from build123d import *
from OCP.BRepFilletAPI import BRepFilletAPI_MakeChamfer

# Parameters (mm, degrees)
ESQUISSE1_W             = 20
ESQUISSE1_H             = 34
BOSS_EXTRU_1_DEPTH      = 4
ESQUISSE2_W             = 8
ESQUISSE2_H             = 7
ENL_V_MAT_EXTRU_1_DEPTH = 21.124611797
CONG_1_R                = 4
ESQUISSE3_W             = 6
ESQUISSE3_H             = 34
BOSS_EXTRU_2_DEPTH      = 20
ESQUISSE4_R             = 2.1
ENL_V_MAT_EXTRU_2_DEPTH = 36.566838488
CHANFREIN1_SIZE         = 8
CHANFREIN1_SIZE2        = 4.618802154
CONG_2_R                = 4
ESQUISSE5_R             = 3.2
ENL_V_MAT_EXTRU_3_DEPTH = 29.08914381
ESQUISSE6_R             = 5.5
ENL_V_MAT_EXTRU_4_DEPTH = 29.08914381
ESQUISSE7_R             = 4
ENL_V_MAT_EXTRU_5_DEPTH = 3


with BuildPart() as part:
    # Esquisse1 → Boss.-Extru.1 (new body)
    with BuildSketch(Plane.XY):
        Rectangle(ESQUISSE1_W, ESQUISSE1_H)
    extrude(amount=BOSS_EXTRU_1_DEPTH)

    # Esquisse2 → Enlèv. mat.-Extru.1 (cut, through all)
    with BuildSketch(Plane.XY.offset(4)):
        with Locations((0, 13.5)):
            Rectangle(ESQUISSE2_W, ESQUISSE2_H)
        with Locations((0, -13.5)):
            Rectangle(ESQUISSE2_W, ESQUISSE2_H)
    extrude(amount=-ENL_V_MAT_EXTRU_1_DEPTH, mode=Mode.SUBTRACT)

    # Congé1
    cong_1_edges = [part.edges().sort_by_distance(p)[0] for p in [
        (0, -10, 4),
        (0, 10, 4),
    ]]
    fillet(cong_1_edges, radius=CONG_1_R - 0.0001)  # a hair under: the kernel refuses the full size

    # Esquisse3 → Boss.-Extru.2 (add)
    with BuildSketch(Plane.XY.offset(4)):
        with Locations((-7, 0)):
            Rectangle(ESQUISSE3_W, ESQUISSE3_H)
        with Locations((7, 0)):
            Rectangle(ESQUISSE3_W, ESQUISSE3_H)
    extrude(amount=BOSS_EXTRU_2_DEPTH)

    # Esquisse4 → Enlèv. mat.-Extru.2 (cut, through all)
    with BuildSketch(Plane(origin=(10, 0, 0), x_dir=(0, 0, -1), z_dir=(1, 0, 0))):
        with Locations(Location((-19, 9, 0), (0, 0, 90))):
            Circle(ESQUISSE4_R)
        with Locations(Location((-19, -9, 0), (0, 0, 90))):
            Circle(ESQUISSE4_R)
    extrude(amount=-ENL_V_MAT_EXTRU_2_DEPTH, mode=Mode.SUBTRACT)

    # Chanfrein1: one chamfer whose edges measure the first distance from different faces: ONE call of the kernel's chamfer builder (chamfer() names one face for all edges)
    chanfrein1_edges_1 = [part.edges().sort_by_distance(p)[0] for p in [
        (-7, -17, 24),
    ]]
    chanfrein1_side_1 = [part.faces().sort_by_distance(p)[0] for p in [
        (-7, -17, 12),
    ]]
    chanfrein1_edges_2 = [part.edges().sort_by_distance(p)[0] for p in [
        (-7, 17, 24),
    ]]
    chanfrein1_side_2 = [part.faces().sort_by_distance(p)[0] for p in [
        (-7, 17, 12),
    ]]
    chanfrein1_edges_3 = [part.edges().sort_by_distance(p)[0] for p in [
        (7, -17, 24),
    ]]
    chanfrein1_side_3 = [part.faces().sort_by_distance(p)[0] for p in [
        (7, -17, 12),
    ]]
    chanfrein1_edges_4 = [part.edges().sort_by_distance(p)[0] for p in [
        (7, 17, 24),
    ]]
    chanfrein1_side_4 = [part.faces().sort_by_distance(p)[0] for p in [
        (7, 17, 12),
    ]]
    chanfrein1 = BRepFilletAPI_MakeChamfer(part.part.solid().wrapped)
    for e in chanfrein1_edges_1:
        chanfrein1.Add(CHANFREIN1_SIZE, CHANFREIN1_SIZE2, e.wrapped, chanfrein1_side_1[0].wrapped)  # the first distance lies on this face
    for e in chanfrein1_edges_2:
        chanfrein1.Add(CHANFREIN1_SIZE, CHANFREIN1_SIZE2, e.wrapped, chanfrein1_side_2[0].wrapped)  # the first distance lies on this face
    for e in chanfrein1_edges_3:
        chanfrein1.Add(CHANFREIN1_SIZE, CHANFREIN1_SIZE2, e.wrapped, chanfrein1_side_3[0].wrapped)  # the first distance lies on this face
    for e in chanfrein1_edges_4:
        chanfrein1.Add(CHANFREIN1_SIZE, CHANFREIN1_SIZE2, e.wrapped, chanfrein1_side_4[0].wrapped)  # the first distance lies on this face
    add(Compound.cast(chanfrein1.Shape()), mode=Mode.REPLACE)

    # Congé2
    cong_2_edges = [part.edges().sort_by_distance(p)[0] for p in [
        (-7, 12.381197846, 24),
        (-7, -12.381197846, 24),
        (-7, -17, 16),
        (7, 12.381197846, 24),
        (7, -12.381197846, 24),
        (7, -17, 16),
        (-7, 17, 16),
        (7, 17, 16),
    ]]
    fillet(cong_2_edges, radius=CONG_2_R)

    # Esquisse5 → Enlèv. mat.-Extru.3 (cut, through all)
    with BuildSketch(Plane.XY.offset(4)):
        Circle(ESQUISSE5_R)
    extrude(amount=-ENL_V_MAT_EXTRU_3_DEPTH, mode=Mode.SUBTRACT)

    # Esquisse6 → Enlèv. mat.-Extru.4 (cut, through all)
    with BuildSketch(Plane.XY.offset(4)):
        Circle(ESQUISSE6_R)
    extrude(amount=ENL_V_MAT_EXTRU_4_DEPTH, mode=Mode.SUBTRACT)

    # Esquisse7 → Enlèv. mat.-Extru.5 (cut)
    with BuildSketch(Plane(origin=(10, 0, 0), x_dir=(0, 0, -1), z_dir=(1, 0, 0))):
        with Locations(Location((-19, 9, 0), (0, 0, 90))):
            Circle(ESQUISSE7_R)
        with Locations(Location((-19, -9, 0), (0, 0, 90))):
            Circle(ESQUISSE7_R)
    extrude(amount=-ENL_V_MAT_EXTRU_5_DEPTH, mode=Mode.SUBTRACT)


solid = part.part
Geometry check sheet. Reference: the model listing, model coordinates, mm. A direction names the side the tool comes from. Round coordinates to 2 decimals unless told otherwise and drop trailing zeros. Write each loop counter-clockwise with the first axis right and the second up, starting at its lowest first coordinate (ties: lowest second). Pieces come first, ordered by that corner, then holes. Notation, with made-up numbers: (-32, 46) -> (4, 46) arc R21 ccw to (4, 64) -> close; hole circle Ø5 at (47, -30.75). An arc over 180 degrees is marked (long way). One line per item, written item: value. Start each with the question number.
(1) Scan lines: line 1 (X direction, y = 8, z = 6.75); line 2 (Z direction, x = 8.55, y = -9); line 3 (X direction, y = -11.5, z = 21). Record each from-to range of solid material in increasing order. Write a range as [from, to].
(2) Go/stop test with flat-tipped pins: pin 1 Ø4 at (y, z) = (-9, 19.5) entering from +X; pin 2 Ø3 at (x, z) = (-2, 3) entering from -Y; pin 3 Ø4 at (x, z) = (-1.5, 19) entering from -Y; pin 4 Ø8.5 at (x, y) = (0, 0) entering from +Z. Record where each tip stops, or that it passes through.
(3) Cross-section at D-D, the plane y = 9. Record the cut outline in (x, z), and give its area (3 significant figures).
(4) Access from +Z, -Z, +X, -X, +Y, -Y to the whole of each face (thin tool, end or side, straight path). Record for faces 1 (the cylindrical face through (7.042, -12.046, 23.479)), 2 (the flat face through (7, 11, 17)).
(5) Cross-section at A-A, the plane z = 5. Record the cut outline in (x, y), and give its area (3 significant figures).
(6) Cross-section at C-C, the plane y = 0. Record the cut outline in (x, z).
(7) Draft check along Y on faces 3 (the flat face through (7, 17, 7)), 4 (the flat face through (6.96, -14.98, 19.5)), 5 (the cylindrical face through (-5.5, 0.1, 13.9)), 6 (the cylindrical face through (-6.958, -10.548, 20.419)). Enter one of: +Y half, -Y half, draft (parallel to the pull), parting line (faces both ways), or undercut.
Answer:
1. line 1: [-10, -4], [4, 10]
1. line 2: [0, 15], [23, 24]
1. line 3: [-10, -4], [4, 7]
2. pin 1: x = 7
2. pin 2: y = -9.71
2. pin 3: through
2. pin 4: z = 4
3. outline: (-10, 0) -> (10, 0) -> (10, 15) -> (7, 15) -> (7, 16.9) -> (4, 16.9) -> (4, 2.65) -> (-4, 2.65) -> (-4, 16.9) -> (-10, 16.9) -> close; (-10, 21.1) -> (-4, 21.1) -> (-4, 24) -> (-10, 24) -> close; (4, 21.1) -> (7, 21.1) -> (7, 23) -> (10, 23) -> (10, 24) -> (4, 24) -> close
3. area: 247 mm²
4. face 1: +Z, +X, -X, -Y
4. face 2: +X
5. outline: (-10, -17) -> (-4, -17) -> (-4, -3.77) arc R5.5 cw to (-4, 3.77) -> (-4, 17) -> (-10, 17) -> close; (4, -17) -> (10, -17) -> (10, 17) -> (4, 17) -> (4, 3.77) arc R5.5 cw to (4, -3.77) -> close
5. area: 392 mm²
6. outline: (-10, 0) -> (-3.2, 0) -> (-3.2, 4) -> (-5.5, 4) -> (-5.5, 24) -> (-10, 24) -> close; (3.2, 0) -> (10, 0) -> (10, 24) -> (5.5, 24) -> (5.5, 4) -> (3.2, 4) -> close
7. face 3: +Y half
7. face 4: -Y half
7. face 5: undercut
7. face 6: undercut
